Design review of the part built by this model. Coordinates are the model's own, in mm. Face numbers are marked on the shaded views. Give positions to 0.01 mm unless a question says otherwise; leave off trailing zeros.
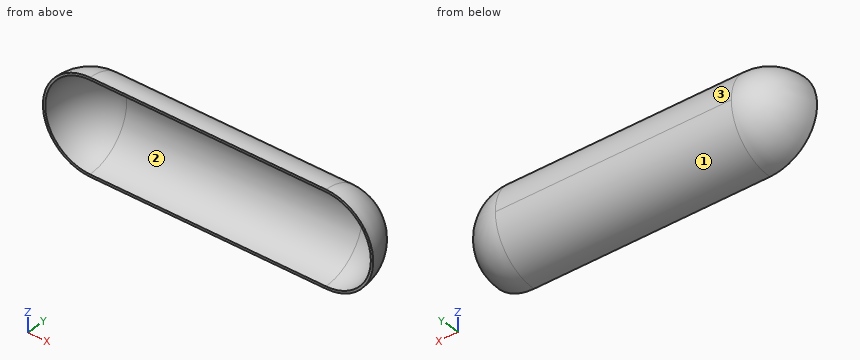
```python
from build123d import *

# Parameters (mm, degrees)
BOSS_EXTRUDE1_DEPTH = 10
FILLET1_R           = 10


# Read off the part's stored shape, not the designer's step: Shell1
with BuildPart() as part:
    # Sketch1 → Boss-Extrude1 (new body)
    with BuildSketch(Plane(origin=(0, 0, 0), x_dir=(1, 0, 0), z_dir=(0, 1, 0))):
        with BuildLine():
            Line((-25, 10), (25, 10))
            ThreePointArc((25, 10), (35, 0), (25, -10))
            Line((25, -10), (-25, -10))
            ThreePointArc((-25, -10), (-35, 0), (-25, 10))
        make_face()
    extrude(amount=BOSS_EXTRUDE1_DEPTH)

    # Fillet1
    fillet1_edges = [part.edges().sort_by_distance(p)[0] for p in [
        (-35, 10, 0),
        (0, 10, -10),
        (35, 10, 0),
        (0, 10, 10),
    ]]
    fillet(fillet1_edges, radius=FILLET1_R - 0.0001)  # a hair under: the kernel refuses the full size

    # Shell1 outline → Shell1 (revolve, cut)
    with BuildSketch(Plane.YX):
        with BuildLine():
            Line((9.5, -25), (9.5, 25))
            ThreePointArc((9.5, 25), (6.717514421, 31.717514421), (0, 34.5))
            Line((0, 34.5), (0, -34.5))
            ThreePointArc((0, -34.5), (6.717514421, -31.717514421), (9.5, -25))
        make_face()
    revolve(axis=Axis((0, 0, 0), (1, 0, 0)), mode=Mode.SUBTRACT)


solid = part.part
```
(1) To check wall thickness, follow L1, parallel to Z at x = -17, y = 0.5; L2, parallel to X at y = 1, z = -7.5. State the ranges of each line that lie inside material, in increasing order.
Resolved:
L1: z = -9.99 to -9.49, 9.49 to 9.99
L2: x = -31.54 to -30.74, 30.74 to 31.54
(2) Clearance check with flat-ended pins moving along their axes: P1, Ø5, axis at y = 4, z = -1.5, coming from the -X side; P2, Ø1, axis at y = 8, z = -3.5, coming from the -X side; P3, Ø3, axis at x = -15, z = 4, coming from the -Y side. State where each tip first meets the part, or that it passes through.
Resolved:
P1: stops at x = -34.84
P2: stops at x = -30.68
P3: stops at y = 7.75
(3) Mouldability with a two-part tool opening along Z and no side actions: class the marked faces 1, 2 and 3 as pulls with the +Z half, pulls with the -Z half, needs draft (parallel to the pull), parting line crosses it, or undercut.
Resolved:
face 1: pulls with the -Z half
face 2: undercut
face 3: pulls with the +Z half
